Read the model definition and answer for the solid it produces. Units are mm, in the model's axes. Coordinates: 2 decimals unless noted, no trailing zeros. Write each loop counter-clockwise with the first axis right and the second up, starting at its lowest first coordinate (ties: lowest second). Pieces come first, ordered by that corner, then holes. Notation, with made-up numbers: M -17.75,-3 L 15.25,-3 A15 ccw 15.25,16 Z; hole C -11,79 d4. An arc over 180 degrees is marked long. Write item = value, one per line.
from build123d import *

# Parameters (mm, degrees)
F0_R     = 71
F1_DEPTH = 60


with BuildPart() as f1:
    # F0 (on Front) → F1 (new body)
    with BuildSketch(Plane.XZ):
        with BuildLine():
            ThreePointArc((-813.985563, 103.535805), (-222.842293, 678.27021), (355.920681, 91.070567))
            Line((355.920681, 91.070567), (800.901331, 86.329341))
            ThreePointArc((800.901331, 86.329341), (-218.10113, 1123.244952), (-1258.966213, 108.277031))
            Line((-1258.966213, 108.277031), (-813.985563, 103.535805))
        make_face()
        with Locations((-1139.994805, 222.242215)):
            Circle(F0_R, mode=Mode.SUBTRACT)
        with Locations((-1075.58415, 453.612111)):
            Circle(F0_R, mode=Mode.SUBTRACT)
        with Locations((684.177669, 204.521474)):
            Circle(F0_R, mode=Mode.SUBTRACT)
        with Locations((624.273984, 437.099009)):
            Circle(F0_R, mode=Mode.SUBTRACT)
        with Locations((-953.485299, 660.427565)):
            Circle(F0_R, mode=Mode.SUBTRACT)
        with Locations((-782.019088, 828.594444)):
            Circle(F0_R, mode=Mode.SUBTRACT)
        with Locations((-572.870654, 946.652456)):
            Circle(F0_R, mode=Mode.SUBTRACT)
        with Locations((-340.293119, 1006.55614)):
            Circle(F0_R, mode=Mode.SUBTRACT)
        with Locations((506.215973, 646.247443)):
            Circle(F0_R, mode=Mode.SUBTRACT)
        with Locations((338.049093, 817.713654)):
            Circle(F0_R, mode=Mode.SUBTRACT)
        with Locations((131.233639, 939.812505)):
            Circle(F0_R, mode=Mode.SUBTRACT)
        with Locations((-100.136257, 1004.22316)):
            Circle(F0_R, mode=Mode.SUBTRACT)
    extrude(amount=F1_DEPTH)


solid = f1.part
Item 1: Find section D-D (z = 476). Determine the outline of the cut face in (x, y).
Worked answers:
outline = M -1185.34,-60 L -1142.96,-60 L -1142.96,0 L -1185.34,0 Z; M -1008.21,-60 L -671.53,-60 L -671.53,0 L -1008.21,0 Z; M 213.38,-60 L 564.88,-60 L 564.88,0 L 213.38,0 Z; M 683.67,-60 L 727.19,-60 L 727.19,0 L 683.67,0 Z
Item 2: Find section B-B (x = -98.5). Determine the outline of the cut face in (y, z).
Worked answers:
outline = M -60,663.54 L 0,663.54 L 0,933.24 L -60,933.24 Z; M -60,1075.2 L 0,1075.2 L 0,1114.99 L -60,1114.99 Z
Item 3: For a pull along Z with two mould halves and no side action, classify faces 1 (the face through (-243, 0, 727)), 2 (the face through (-625.2, -29.58, 994.64)) as released by +Z, released by -Z, zero draft, split by the parting line, or undercut.
Worked answers:
face_1 = zero draft
face_2 = undercut
Item 4: Flat-ended cylindrical pins translate along their axes: pin 1 (12 mm diameter, centred on x = 189, y = -44, fed in from -Z); pin 2 (5 mm diameter, centred on x = -278, z = 768.5, fed in from +Y); pin 3 (8 mm diameter, centred on x = -520.5, y = -29, fed in from +Z); pin 4 (6 mm diameter, centred on y = -39, z = 837.5, fed in from +X). Find the tip coordinate at first contact, or state that the pin passes through.
Worked answers:
pin_1 = 496.27
pin_2 = 0
pin_3 = 1082.39
pin_4 = 486.14
Item 5: Consider line 1 along X through (y, z) = (-20.5, 966); line 2 along X through (y, z) = (-26, 613); line 3 along X through (y, z) = (-49, 148). Determine where each line is inside the solid, lowest interval first. Write a range as from..to.
Worked answers:
line_1 = -776.16..-641.18, -504.56..-398.57, -282.02..-159.97, -40.3..65.24, 197.23..318.01
line_2 = -1118.35..-1006.32, -900.65..-497.66, 39.51..443.48, 568.95..660.2
line_3 = -1257.62..-811.51, 353.36..641.21, 727.15..799.47
Item 6: Find section A-A (z = 248.5). Determine the outline of the cut face in (x, y).
Worked answers:
outline = M -1247.32,-60 L -1205.96,-60 L -1205.96,0 L -1247.32,0 Z; M -1074.03,-60 L -793.11,-60 L -793.11,0 L -1074.03,0 Z; M 334.96,-60 L 628.44,-60 L 628.44,0 L 334.96,0 Z; M 739.92,-60 L 789.17,-60 L 789.17,0 L 739.92,0 Z
Item 7: Find section C-C (y = -42.5). State how many separate pieces and enclosed holes the cut face has, and give its area (3 significant figures).
Worked answers:
separate_pieces = 1
enclosed_holes = 12
area = 935,000 mm²
